Print and shaded views of the part. All mm, measured from the part's lowest x, y and z. Coordinates: 2 decimals unless noted, no trailing zeros. Loops run counter-clockwise (first coordinate to the right, second up) from the corner with the lowest first, then second, coordinate; pieces in that order, holes last.
1) Saw through at A-A, the plane y = 7.5. Write the cut outline in (x, z) (3 decimals).
2) Saw through at B-B, the plane x = 0.9. Write the cut outline in (y, z) (3 decimals).
3) Wall check: line 1 along Y through (x, z) = (0.8, 4.5); line 2 along Y through (x, z) = (0.65, 5). Give the ranges that are in metal, low to high.
4) Pin check, flat tip, straight feed: pin 1 Ø0.8 at (x, y) = (0.5, 8) entering from -Z. Stop position of the tip, or through.
5) Saw through at C-C, the plane y = 9.5. Write the cut outline in (x, z), and give its area (3 significant figures).
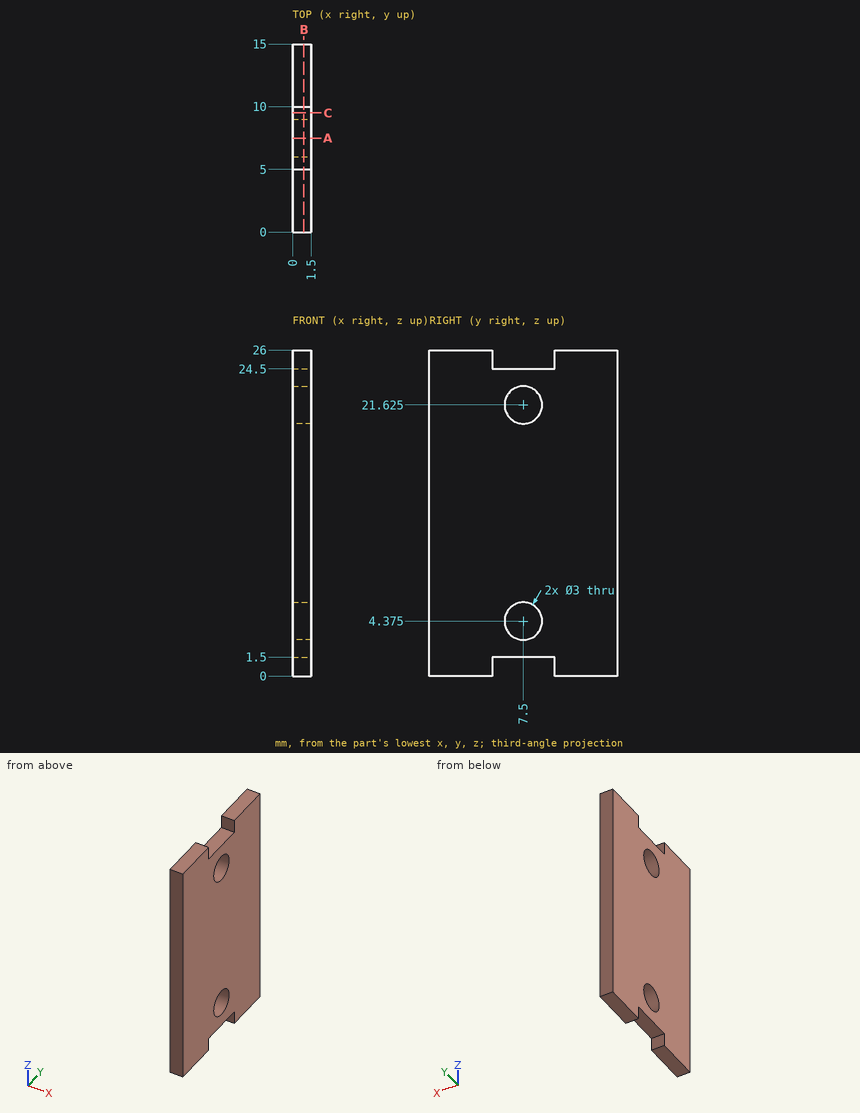
Data:
1. outline: (0, 1.5) - (1.5, 1.5) - (1.5, 2.875) - (0, 2.875) - close; (0, 5.875) - (1.5, 5.875) - (1.5, 20.125) - (0, 20.125) - close; (0, 23.125) - (1.5, 23.125) - (1.5, 24.5) - (0, 24.5) - close
2. outline: (0, 0) - (5, 0) - (5, 1.5) - (10, 1.5) - (10, 0) - (15, 0) - (15, 26) - (10, 26) - (10, 24.5) - (5, 24.5) - (5, 26) - (0, 26) - close; hole circle Ø3 at (7.5, 4.375); hole circle Ø3 at (7.5, 21.625)
3. line 1: y = 0 to 6.01, 8.99 to 15
3. line 2: y = 0 to 6.14, 8.86 to 15
4. pin 1: stops at z = 1.5
5. outline: (0, 1.5) - (1.5, 1.5) - (1.5, 24.5) - (0, 24.5) - close
5. area: 34.5 mm2
